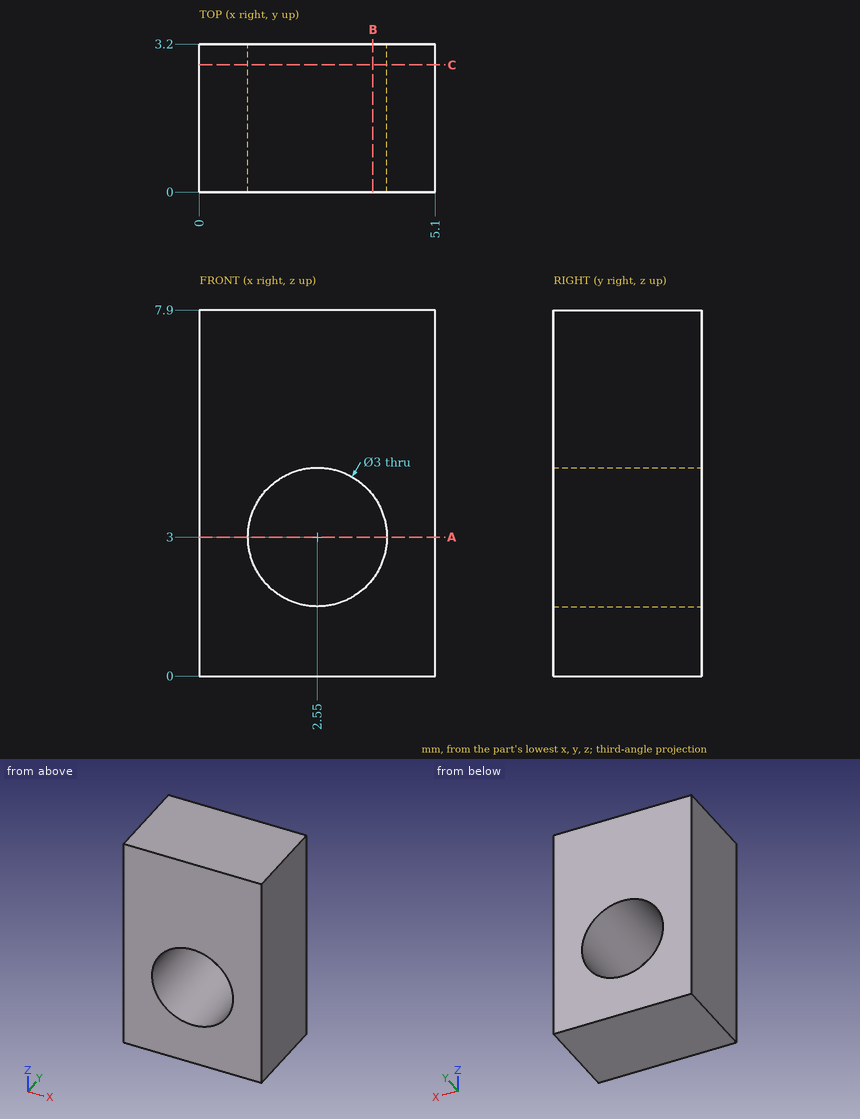
Here's the drawing with two shaded views (mm, measured from the low corner). I have some questions. Give positions to 0.01 mm unless a question says otherwise; leave off trailing zeros. Order: outer loops, then holes, each group sorted by start corner. A loop starts at its lowest first (then second) coordinate and runs counter-clockwise, first axis right, second up.
Q1. Suppose I cut it at B-B, the plane x = 3.75. Write out the boundary of the cut face in (y, z).
Q2. Suppose I cut it at C-C, the plane y = 2.75. Write out the boundary of the cut face in (x, z).
Q3. Suppose I cut it at A-A, the plane z = 3. Write out the boundary of the cut face in (x, y).
Q4. If I drill on line 1 along X through (y, z) = (1.85, 3); line 2 along Z through (x, y) = (2.55, 1.25); line 3 along X through (y, z) = (0.7, 4), over which ranges is the centre line in solid material (lowest first)?
Q5. I'm going to push a flat-ended pin straight in: P1, Ø2.5, axis at x = 2.55, z = 3, coming from the -Y side. Where does the tip first touch, or does it pass through?
Solution:
1. outline: (0, 0) - (3.2, 0) - (3.2, 2.1) - (0, 2.1) - close; (0, 3.9) - (3.2, 3.9) - (3.2, 7.9) - (0, 7.9) - close
2. outline: (0, 0) - (5.1, 0) - (5.1, 7.9) - (0, 7.9) - close; hole circle Ø3 at (2.55, 3)
3. outline: (0, 0) - (1.05, 0) - (1.05, 3.2) - (0, 3.2) - close; (4.05, 0) - (5.1, 0) - (5.1, 3.2) - (4.05, 3.2) - close
4. line 1: x = 0 to 1.05, 4.05 to 5.1
4. line 2: z = 0 to 1.5, 4.5 to 7.9
4. line 3: x = 0 to 1.43, 3.67 to 5.1
5. P1: passes through
